For this review, take the finished solid that the model builds, in its own axes (mm). Face numbers are marked on the shaded views. Coordinates: 2 decimals unless noted, no trailing zeros. Order: outer loops, then holes, each group sorted by start corner. A loop starts at its lowest first (then second) coordinate and runs counter-clockwise, first axis right, second up. Notation, with made-up numbers: (-31, 55.5) -> (28, 55.5) arc R12 ccw to (28, 60.5) -> close; hole circle Ø7 at (60, -33). An arc over 180 degrees is marked (long way). Return JSON: item names as keys, results as strings. Group by question number.
Item 1: Take a section at D-D (x = 21). Write out the cut boundary in (y, z), then the cut area to 3 significant figures.
Item 2: Take a section at C-C (y = -6). Write out the cut boundary in (x, z).
Item 3: Insertion check: pin 1 (1 mm diameter, centred on y = 11, z = 42.5, fed in from +X); pin 2 (2 mm diameter, centred on y = 29.5, z = 72, fed in from +X); pin 3 (6 mm diameter, centred on x = 4.5, y = 38, fed in from +Z); pin 4 (12 mm diameter, centred on x = -5.5, z = 68.5, fed in from +Y). Each pin has a flat end and moves straight along its axis. Give the tip position at first contact, or say it passes through.
Item 4: For line 1 along Z through (x, y) = (0, 41); line 2 along Y through (x, z) = (0, 68); line 3 along X through (y, z) = (24.5, 37), list the stretches that pass through material, from the lowest coordinate up.
Item 5: Take a section at B-B (z = 50.8). Write out the cut boundary in (x, y).
Item 6: Draft analysis for pull direction Z (two halves, no side actions). For the marked faces 1, 2 and 3, state which applies: +Z half, -Z half, draft (parallel to the pull), parting line (faces both ways), or undercut.
Item 7: Take a section at A-A (x = 0). Write out the cut boundary in (y, z).
```python
from build123d import *

# Parameters (mm, degrees)
SKETCH1_R           = 24.13
SKETCH1_R_2         = 19.05
BOSS_EXTRUDE1_DEPTH = 101.6
SKETCH2_R           = 24.13
SKETCH2_R_2         = 19.05
BOSS_EXTRUDE2_DEPTH = 50.8
SKETCH3_R           = 19.05
CUT_EXTRUDE1_DEPTH  = 102.6000001


with BuildPart() as part:
    # Sketch1 → Boss-Extrude1 (new body)
    with BuildSketch(Plane.XY):
        Circle(SKETCH1_R)
        Circle(SKETCH1_R_2, mode=Mode.SUBTRACT)
    extrude(amount=BOSS_EXTRUDE1_DEPTH)

    # Sketch2 → Boss-Extrude2 (add)
    with BuildSketch(Plane(origin=(0, 0, 0), x_dir=(1, 0, 0), z_dir=(0, 1, 0))):
        with Locations((0, -50.8)):
            Circle(SKETCH2_R)
        with Locations((0, -50.8)):
            Circle(SKETCH2_R_2, mode=Mode.SUBTRACT)
    extrude(amount=BOSS_EXTRUDE2_DEPTH)

    # Sketch3 → Cut-Extrude1 (cut, through all)
    with BuildSketch(Plane.XY.offset(101.6)):
        Circle(SKETCH3_R)
    extrude(amount=-CUT_EXTRUDE1_DEPTH, mode=Mode.SUBTRACT)


solid = part.part
```
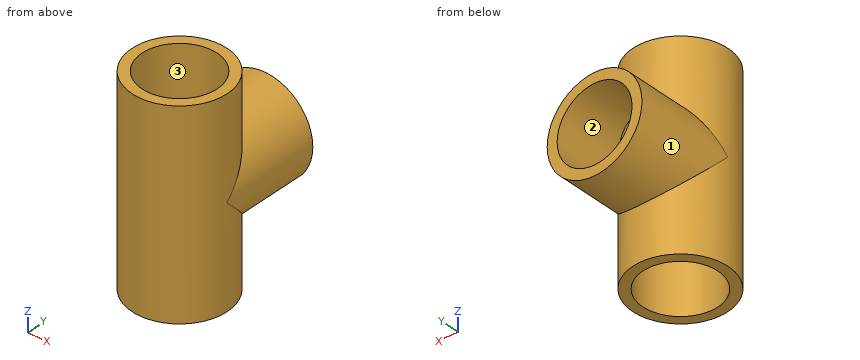
Findings below:
{
 "1": {"outline": "(-11.89, 0) -> (11.89, 0) -> (11.89, 38.91) -> (50.8, 38.91) -> (50.8, 62.69) -> (11.89, 62.69) -> (11.89, 101.6) -> (-11.89, 101.6) -> close", "area": "3,340 mm2"},
 "2": {"outline": "(-23.37, 0) -> (-18.08, 0) -> (-18.08, 101.6) -> (-23.37, 101.6) -> close; (18.08, 0) -> (23.37, 0) -> (23.37, 101.6) -> (18.08, 101.6) -> close"},
 "3": {"pin 1": "stops at x = 22.83", "pin 2": "stops at x = 13.2", "pin 3": "stops at z = 74.88", "pin 4": "stops at y = 50.8"},
 "4": {"line 1": "z = 26.67 to 31.75, 69.85 to 74.93", "line 2": "y = -24.13 to -19.05, 19.05 to 24.13", "line 3": "x = -19.79 to -13.13, 13.13 to 19.79"},
 "5": {"outline": "(-24.13, 0) arc R24.13 ccw to (24.13, 0) -> (24.13, 50.8) -> (19.05, 50.8) -> (19.05, 14.81) arc R24.13 ccw to (-19.05, 14.81) -> (-19.05, 50.8) -> (-24.13, 50.8) -> close; hole circle Ø38.1 at (0, 0)"},
 "6": {"face 1": "parting line", "face 2": "undercut", "face 3": "draft"},
 "7": {"outline": "(-24.13, 0) -> (-19.05, 0) -> (-19.05, 101.6) -> (-24.13, 101.6) -> close; (19.05, 0) -> (24.13, 0) -> (24.13, 26.67) -> (50.8, 26.67) -> (50.8, 31.75) -> (24.13, 31.75) -> (24.13, 69.85) -> (50.8, 69.85) -> (50.8, 74.93) -> (24.13, 74.93) -> (24.13, 101.6) -> (19.05, 101.6) -> close"}
}
